Source: CAD feature listing. Evaluate the final solid. Frame: model axes, mm. A direction names the side the tool comes from. Coordinates: 2 decimals unless noted, no trailing zeros. Write each loop counter-clockwise with the first axis right and the second up, starting at its lowest first coordinate (ties: lowest second). Pieces come first, ordered by that corner, then holes. Notation, with made-up numbers: (-24, 78.5) - (-20, 78.5) arc R16 cw to (-20, 99.5) - close; hole circle Ø8 at (14, 68.5). An arc over 180 degrees is marked (long way). One line per item, written item: value.
from build123d import *

# Parameters (mm, degrees)
SKETCH1_W           = 48.514
SKETCH1_H           = 48.514
SKETCH1_R           = 3.6195
BOSS_EXTRUDE1_DEPTH = 12.7
FILLET1_R           = 3.81
SKETCH4_R           = 5.715
CUT_EXTRUDE2_DEPTH  = 5.08
BOSS_EXTRUDE3_DEPTH = 26.67
SKETCH8_R           = 13.12545
CUT_EXTRUDE4_DEPTH  = 7.762
SKETCH11_W          = 6.238
SKETCH11_H          = 6.238
CUT_EXTRUDE7_DEPTH  = 68.022437624
SKETCH13_W          = 5.08
SKETCH13_H          = 6.238
CUT_EXTRUDE8_DEPTH  = 55.130822948
SKETCH14_W          = 10.16
SKETCH14_H          = 6.238
BOSS_EXTRUDE4_DEPTH = 1.016
FILLET3_R           = 5.08
FILLET2_R           = 2.54
FILLET4_R           = 2.032
FILLET6_R           = 5.08


# Some blends are built 0.0001 mm under size
with BuildPart() as part:
    # Sketch1 → Boss-Extrude1 (new body)
    with BuildSketch(Plane(origin=(0, 0, 0), x_dir=(1, 0, 0), z_dir=(0, 1, 0))):
        Rectangle(SKETCH1_W, SKETCH1_H)
        with Locations(Location((-17.907, 17.907, 0), (0, 0, 270))):
            Circle(SKETCH1_R, mode=Mode.SUBTRACT)
        with Locations(Location((17.907, 17.907, 0), (0, 0, 270))):
            Circle(SKETCH1_R, mode=Mode.SUBTRACT)
        with Locations(Location((17.907, -17.907, 0), (0, 0, 270))):
            Circle(SKETCH1_R, mode=Mode.SUBTRACT)
        with Locations(Location((-17.907, -17.907, 0), (0, 0, 270))):
            Circle(SKETCH1_R, mode=Mode.SUBTRACT)
    extrude(amount=BOSS_EXTRUDE1_DEPTH)

    # Fillet1
    fillet1_edges = [part.edges().sort_by_distance(p)[0] for p in [
        (24.257, 6.35, 24.257),
        (-24.257, 6.35, 24.257),
        (-24.257, 6.35, -24.257),
        (24.257, 6.35, -24.257),
    ]]
    fillet(fillet1_edges, radius=FILLET1_R)

    # Sketch4 → Cut-Extrude2 (cut)
    with BuildSketch(Plane(origin=(0, 12.7, 0), x_dir=(1, 0, 0), z_dir=(0, 1, 0))):
        with Locations(Location((-17.907, 17.907, 0), (0, 0, 270))):
            Circle(SKETCH4_R)
        with Locations(Location((17.907, -17.907, 0), (0, 0, 270))):
            Circle(SKETCH4_R)
        with Locations(Location((17.907, 17.907, 0), (0, 0, 270))):
            Circle(SKETCH4_R)
        with Locations(Location((-17.907, -17.907, 0), (0, 0, 270))):
            Circle(SKETCH4_R)
    extrude(amount=-CUT_EXTRUDE2_DEPTH, mode=Mode.SUBTRACT)

    # Sketch6 → Boss-Extrude3 (add)
    with BuildSketch(Plane(origin=(0, 12.7, 0), x_dir=(1, 0, 0), z_dir=(0, 1, 0))):
        Polygon((-3.881, 17.907), (-3.881, -17.907), (-9.525, -17.907), (-9.525, -24.257), (9.525, -24.257), (9.525, -17.907), (3.881, -17.907), (3.881, 17.907), (9.525, 17.907), (9.525, 24.257), (-9.525, 24.257), (-9.525, 17.907), align=None)
    extrude(amount=BOSS_EXTRUDE3_DEPTH)

    # Sketch8 → Cut-Extrude4 (cut)
    with BuildSketch(Plane(origin=(3.881, 0, 0), x_dir=(0, 0, -1), z_dir=(1, 0, 0))):
        with Locations((0, 39.37)):
            Circle(SKETCH8_R)
    extrude(amount=-CUT_EXTRUDE4_DEPTH, mode=Mode.SUBTRACT)

    # Sketch11 → Cut-Extrude7 (cut, through all)
    with BuildSketch(Plane.XY.offset(24.257)):
        with Locations((0, 20.58555)):
            Rectangle(SKETCH11_W, SKETCH11_H)
    extrude(amount=-CUT_EXTRUDE7_DEPTH, mode=Mode.SUBTRACT)

    # Sketch13 → Cut-Extrude8 (cut, through all)
    with BuildSketch(Plane(origin=(3.881, 0, 0), x_dir=(0, 0, -1), z_dir=(1, 0, 0))):
        with Locations((-2.54, 20.58555)):
            Rectangle(SKETCH13_W, SKETCH13_H)
        with Locations((2.54, 20.58555)):
            Rectangle(SKETCH13_W, SKETCH13_H)
    extrude(amount=-CUT_EXTRUDE8_DEPTH, mode=Mode.SUBTRACT)

    # Sketch14 → Boss-Extrude4 (add)
    with BuildSketch(Plane(origin=(3.881, 0, 0), x_dir=(0, 0, -1), z_dir=(1, 0, 0))):
        with BuildLine():
            Line((17.907, 39.37), (8.04545, 39.37))
            ThreePointArc((8.04545, 39.37), (0, 31.32455), (-8.04545, 39.37))
            Line((-8.04545, 39.37), (-17.907, 39.37))
            Line((-17.907, 39.37), (-17.907, 12.7))
            Line((-17.907, 12.7), (17.907, 12.7))
            Line((17.907, 12.7), (17.907, 39.37))
        make_face()
        with Locations((0, 20.58555)):
            Rectangle(SKETCH14_W, SKETCH14_H, mode=Mode.SUBTRACT)
    boss_extrude4 = extrude(amount=BOSS_EXTRUDE4_DEPTH)

    # Mirror1: Boss-Extrude4 across plane
    add(boss_extrude4.mirror(Plane(origin=(0, 0, 0), x_dir=(0, 0, 1), z_dir=(1, 0, 0))))

    # Fillet3
    fillet3_edges = [part.edges().sort_by_distance(p)[0] for p in [
        (0, 23.70455, -24.257),
        (0, 23.70455, 24.257),
        (0, 39.37, 24.257),
        (0, 39.37, -24.257),
    ]]
    fillet(fillet3_edges, radius=FILLET3_R)

    # Fillet2
    fillet2_edges = [part.edges().sort_by_distance(p)[0] for p in [
        (4.897, 26.035, -17.907),
        (4.897, 26.035, 17.907),
        (-4.897, 26.035, -17.907),
        (-4.897, 26.035, 17.907),
    ]]
    fillet(fillet2_edges, radius=FILLET2_R)

    # Fillet4
    # the kernel refuses this fillet: 2.032 mm, written as the material it adds along each edge
    with BuildSketch(Plane(origin=(3.119, 23.70455, 19.177), x_dir=(-1, 0, 0), z_dir=(0, 0, -1)), Plane(origin=(3.119, 23.70455, -5.08), x_dir=(-1, 0, 0), z_dir=(0, 0, -1))) as fillet4_piece_1:
        with BuildLine():
            CenterArc((FILLET4_R, -FILLET4_R), FILLET4_R, 90, 90)
            Line((0, -FILLET4_R), (0, 0))
            Line((0, 0), (FILLET4_R, 0))
        make_face()
    extrude(amount=14.097)
    with BuildSketch(Plane(origin=(-3.119, 23.70455, 19.177), x_dir=(1, 0, 0), z_dir=(0, 0, -1)), Plane(origin=(-3.119, 23.70455, -5.08), x_dir=(1, 0, 0), z_dir=(0, 0, -1))) as fillet4_piece_2:
        with BuildLine():
            CenterArc((FILLET4_R, FILLET4_R), FILLET4_R, 180, 90)
            Line((0, FILLET4_R), (0, 0))
            Line((0, 0), (FILLET4_R, 0))
        make_face()
    extrude(amount=14.097)
    with BuildSketch(Plane(origin=(-3.119, 28.78455, -19.177), x_dir=(0, 0.8416879607506225, -0.5399642365263265), z_dir=(0, 0.5399642365263265, 0.8416879607506225))) as fillet4_piece_3_section:
        with BuildLine():
            CenterArc((5.08 + FILLET4_R, -FILLET4_R), FILLET4_R, 90, 90)
            Line((5.08, -FILLET4_R), (5.08, 0))
            Line((5.08, 0), (5.08 + FILLET4_R, 0))
        make_face()
    fillet4_piece_3 = revolve(axis=Axis((-3.119, 28.78455, -19.177), (-1, 0, 0)), revolution_arc=147.318795695, mode=Mode.PRIVATE)
    fillet4_piece_3 = split(fillet4_piece_3, bisect_by=Plane(origin=(-3.119, 28.78455, -24.257), z_dir=(0, 0, 1)), keep=Keep.TOP, mode=Mode.PRIVATE)
    add(fillet4_piece_3)
    with BuildSketch(Plane(origin=(3.119, 28.78455, -19.177), x_dir=(0, 0.8416879607506221, -0.5399642365263271), z_dir=(0, 0.5399642365263271, 0.8416879607506221))) as fillet4_piece_4_section:
        with BuildLine():
            CenterArc((5.08 + FILLET4_R, FILLET4_R), FILLET4_R, 180, 90)
            Line((5.08 + FILLET4_R, 0), (5.08, 0))
            Line((5.08, 0), (5.08, FILLET4_R))
        make_face()
    fillet4_piece_4 = revolve(axis=Axis((3.119, 28.78455, -19.177), (-1, 0, 0)), revolution_arc=147.318795695, mode=Mode.PRIVATE)
    fillet4_piece_4 = split(fillet4_piece_4, bisect_by=Plane(origin=(3.119, 28.78455, -24.257), z_dir=(0, 0, 1)), keep=Keep.TOP, mode=Mode.PRIVATE)
    add(fillet4_piece_4)
    with BuildSketch(Plane(origin=(-3.119, 28.78455, 19.177), x_dir=(0, 0.8416879607506225, 0.5399642365263265), z_dir=(0, 0.5399642365263265, -0.8416879607506225))) as fillet4_piece_5_section:
        with BuildLine():
            CenterArc((5.08 + FILLET4_R, FILLET4_R), FILLET4_R, 180, 90)
            Line((5.08, FILLET4_R), (5.08, 0))
            Line((5.08, 0), (5.08 + FILLET4_R, 0))
        make_face()
    fillet4_piece_5 = revolve(axis=Axis((-3.119, 28.78455, 19.177), (1, 0, 0)), revolution_arc=147.318795695, mode=Mode.PRIVATE)
    fillet4_piece_5 = split(fillet4_piece_5, bisect_by=Plane(origin=(-3.119, 28.78455, 24.257), z_dir=(0, 0, -1)), keep=Keep.TOP, mode=Mode.PRIVATE)
    add(fillet4_piece_5)
    with BuildSketch(Plane(origin=(3.119, 28.78455, 19.177), x_dir=(0, 0.8416879607506221, 0.5399642365263271), z_dir=(0, 0.5399642365263271, -0.8416879607506221))) as fillet4_piece_6_section:
        with BuildLine():
            CenterArc((5.08 + FILLET4_R, -FILLET4_R), FILLET4_R, 90, 90)
            Line((5.08, -FILLET4_R), (5.08, 0))
            Line((5.08, 0), (5.08 + FILLET4_R, 0))
        make_face()
    fillet4_piece_6 = revolve(axis=Axis((3.119, 28.78455, 19.177), (1, 0, 0)), revolution_arc=147.318795695, mode=Mode.PRIVATE)
    fillet4_piece_6 = split(fillet4_piece_6, bisect_by=Plane(origin=(3.119, 28.78455, 24.257), z_dir=(0, 0, -1)), keep=Keep.TOP, mode=Mode.PRIVATE)
    add(fillet4_piece_6)

    # Fillet6
    fillet6_edges = [part.edges().sort_by_distance(p)[0] for p in [
        (-2.992, 23.70455, -5.08),
        (2.992, 23.70455, -5.08),
        (-2.992, 23.70455, 5.08),
        (2.992, 23.70455, 5.08),
    ]]
    fillet(fillet6_edges, radius=FILLET6_R - 0.0001)  # a hair under: the kernel refuses the full size


solid = part.part
1) Contact query for flat-ended pins moving along their axis: P1, Ø6, axis at x = -17, z = 0, coming from the +Y side; P2, Ø5, axis at y = 27, z = -2.5, coming from the -X side; P3, Ø5, axis at x = -0.5, y = 22, coming from the -Z side; P4, Ø6.5, axis at x = -17.907, z = -17.907, coming from the -Y side. Output: stop coordinate, or through.
Values found:
P1: y = 12.7
P2: x = -4.9
P3: z = -21.91
P4: through
2) Section query C-C on z = -10. Output: boundary loops of the cut face in (x, y), then the cut area to 3 significant figures.
Values found:
outline: (-24.26, 0) - (24.26, 0) - (24.26, 12.7) - (4.9, 12.7) - (4.9, 39.37) - (3.88, 39.37) - (3.88, 30.87) - (-3.88, 30.87) - (-3.88, 39.37) - (-4.9, 39.37) - (-4.9, 12.7) - (-24.26, 12.7) - close; hole (-3.12, 17.47) - (3.12, 17.47) - (3.12, 21.67) arc R2.03 ccw to (1.09, 23.7) - (-1.09, 23.7) arc R2.03 ccw to (-3.12, 21.67) - close
area: 774 mm2
3) Section query A-A on y = 3.5. Output: boundary loops of the cut face in (x, z).
Values found:
outline: (-24.26, -20.45) arc R3.81 ccw to (-20.45, -24.26) - (20.45, -24.26) arc R3.81 ccw to (24.26, -20.45) - (24.26, 20.45) arc R3.81 ccw to (20.45, 24.26) - (-20.45, 24.26) arc R3.81 ccw to (-24.26, 20.45) - close; hole circle Ø7.24 at (-17.91, -17.91); hole circle Ø7.24 at (-17.91, 17.91); hole circle Ø7.24 at (17.91, -17.91); hole circle Ø7.24 at (17.91, 17.91)
4) Material intervals for line 1 (Z direction, x = 17, y = 4); line 2 (Y direction, x = 20.5, z = -6.5); line 3 (X direction, y = 36, z = -13.5), sorted ascending.
Values found:
line 1: -24.26 to -21.41, -14.4 to 14.4, 21.41 to 24.26
line 2: 0 to 12.7
line 3: -4.9 to 4.9
5) Reachability of faces 1 (the cylindrical face through (2.508, 23.125, 9.723)), 2 (the flat face through (4.897, 26, 0)), 3 (the flat face through (-8, 26, -17.907)) from +Z, -Z, +X, -X, +Y, -Y: full face, straight path, thin tool, end or side. Return the list, or none.
Values found:
face 1: +Z, -Z
face 2: +X, +Y
face 3: -X, +Y
6) Section query D-D on x = 17. Output: boundary loops of the cut face in (y, z).
Values found:
outline: (0, -24.26) - (12.7, -24.26) - (12.7, -23.55) - (7.62, -23.55) - (7.62, -21.41) - (0, -21.41) - close; (0, -14.4) - (7.62, -14.4) - (7.62, -12.26) - (12.7, -12.26) - (12.7, 12.26) - (7.62, 12.26) - (7.62, 14.4) - (0, 14.4) - close; (0, 21.41) - (7.62, 21.41) - (7.62, 23.55) - (12.7, 23.55) - (12.7, 24.26) - (0, 24.26) - close
7) Section query B-B on y = 15. Output: boundary loops of the cut face in (x, z) (3 decimals).
Values found:
outline: (-9.525, -24.257) - (9.525, -24.257) - (9.525, -17.907) - (7.437, -17.907) arc R2.54 cw to (4.897, -15.367) - (4.897, 15.367) arc R2.54 cw to (7.437, 17.907) - (9.525, 17.907) - (9.525, 24.257) - (-9.525, 24.257) - (-9.525, 17.907) - (-7.437, 17.907) arc R2.54 cw to (-4.897, 15.367) - (-4.897, -15.367) arc R2.54 cw to (-7.437, -17.907) - (-9.525, -17.907) - close
8) Draft query along Z for faces 4 (the flat face through (-3.119, 20, -14)), 5 (the cylindrical face through (-0.13, 37.92, -22.73)), 6 (the cylindrical face through (-15.461, 3.757, -20.575)). Return one class per face: released by +Z, released by -Z, zero draft, split by the parting line, or undercut.
Values found:
face 4: zero draft
face 5: released by -Z
face 6: undercut
